```python
from build123d import *

# Parameters (mm, degrees)
SKETCH2_R           = 7.5
BOSS_EXTRUDE1_DEPTH = 5
CHAMFER1_SIZE       = 1
SKETCH3_R           = 5
BOSS_EXTRUDE2_DEPTH = 121
SKETCH4_R           = 2
CUT_EXTRUDE1_DEPTH  = 10


with BuildPart() as part:
    # Sketch2 → Boss-Extrude1 (new body)
    with BuildSketch(Plane.XY):
        Circle(SKETCH2_R)
    extrude(amount=BOSS_EXTRUDE1_DEPTH)

    # Chamfer1
    chamfer1_edges = [part.edges().sort_by_distance(p)[0] for p in [
        (-7.5, 0, 0),
    ]]
    chamfer(chamfer1_edges, length=CHAMFER1_SIZE)

    # Sketch3 → Boss-Extrude2 (add)
    with BuildSketch(Plane.XY.offset(5)):
        Circle(SKETCH3_R)
    extrude(amount=BOSS_EXTRUDE2_DEPTH)

    # Sketch4 → Cut-Extrude1 (cut)
    with BuildSketch(Plane.XY.offset(126)):
        Circle(SKETCH4_R)
    extrude(amount=-CUT_EXTRUDE1_DEPTH, mode=Mode.SUBTRACT)


solid = part.part
```
The listing builds one solid part. Answer for the finished solid, in the listing's coordinates (mm). A direction names the side the tool comes from. Round coordinates to 2 decimals unless told otherwise and drop trailing zeros. Order: outer loops, then holes, each group sorted by start corner. A loop starts at its lowest first (then second) coordinate and runs counter-clockwise, first axis right, second up. Notation, with made-up numbers: (38.25, 15.25) - (68.25, 15.25) arc R26 ccw to (68.25, 30.25) - close; hole circle Ø10 at (60.5, -21.5). An arc over 180 degrees is marked (long way). Put each result on its own line as item: value. Start each with the question number.
(1) Find section C-C (z = 34.5). Give the vertices of the cut face in (x, y).
(2) Find section A-A (y = 0). Give the vertices of the cut face in (x, z).
(3) Straight lines are drawn through the part: probe 1 along Y at (x, z) = (0, 123); probe 2 along Y at (x, z) = (0.5, 17); probe 3 along Z at (x, y) = (-6, -1.25). For each, find the intervals that lie inside material, in ascending order. Write a range as from..to.
(4) Given P1, Ø2, axis at x = 1, y = 0.5, coming from the +Z side; P2, Ø1, axis at x = 3.5, z = 68.5, coming from the +Y side; P3, Ø2, axis at y = 3, z = 54, coming from the -X side; P4, Ø5, axis at x = 1.5, z = 33, coming from the +Y side, each flat-ended and moving along its own axis, determine where each tip first touches the part or whether it passes through.
(5) For faces 1 (the flat face through (2, -5, 5)), 2 (the flat face through (0, 0, 0)), determine the directions among +Z, -Z, +X, -X, +Y, -Y from which every point of the face is accessible in a straight line to the end or side of a thin tool.
(6) Determine the mould class of faces 3 (the flat face through (0, 0, 116)), 4 (the cylindrical face through (-7.493, 0.33, 2.972)), 5 (the flat face through (-0.1, -2.2, 126)) for opening direction X: released by +X, released by -X, zero draft, split by the parting line, or undercut.
Reply:
1. outline: circle Ø10 at (0, 0)
2. outline: (-7.5, 1) - (-6.5, 0) - (6.5, 0) - (7.5, 1) - (7.5, 5) - (5, 5) - (5, 126) - (2, 126) - (2, 116) - (-2, 116) - (-2, 126) - (-5, 126) - (-5, 5) - (-7.5, 5) - close
3. probe 1: -5..-2, 2..5
3. probe 2: -4.97..4.97
3. probe 3: 0..5
4. P1: z = 126
4. P2: y = 4
4. P3: x = -4.58
4. P4: y = 5
5. face 1: +Z
5. face 2: -Z, +X, -X, +Y, -Y
6. face 3: undercut
6. face 4: split by the parting line
6. face 5: zero draft
